from build123d import *

# Parameters (mm, degrees)
CYLINDER692_R               = 8
CYLINDER692_DEPTH           = 25
CYLINDER693_R               = 8
CYLINDER693_DEPTH           = 25
CYLINDER693_PLACEMENT_ANGLE = 225
CYLINDER695_R               = 8
CYLINDER695_DEPTH           = 25
CYLINDER694_R               = 8
CYLINDER694_DEPTH           = 25
CYLINDER694_PLACEMENT_ANGLE = 145
CYLINDER696_R               = 8
CYLINDER696_DEPTH           = 25
CYLINDER697_R               = 8
CYLINDER697_DEPTH           = 25
CYLINDER697_PLACEMENT_ANGLE = 45
CYLINDER690_R               = 8
CYLINDER690_DEPTH           = 25
CYLINDER690_ROLL_ANGLE      = 0.146073
CYLINDER690_PITCH_ANGLE     = 1.079101
CYLINDER690_PLACEMENT_ANGLE = -9.939308
CYLINDER691_R               = 8
CYLINDER691_DEPTH           = 25
CYLINDER691_PLACEMENT_ANGLE = 45
TUBE075_R                   = 38.75
TUBE075_R_2                 = 30
TUBE075_DEPTH               = 8
CHAMFER001_SIZE             = 1


with BuildPart() as obj1:
    # Cylinder692 → Cylinder692 (new body)
    with BuildSketch(Plane(origin=(-38.798949, 16.072537, 43), x_dir=(0, -1, 0), z_dir=(0, 0, 1))):
        Circle(CYLINDER692_R)
    extrude(amount=CYLINDER692_DEPTH)


with BuildPart() as obj2:
    # Cylinder693 → Cylinder693 (new body)
    with BuildSketch(Plane.XY):
        Circle(CYLINDER693_R)
    extrude(amount=CYLINDER693_DEPTH)


with BuildPart() as obj2_1:
    # Cylinder693 placement: moved
    add(obj2.part.moved(Location((-16.07, 38.8, 43))).rotate(Axis((-16.07, 38.8, 43), (0, 0, 1)), CYLINDER693_PLACEMENT_ANGLE))


with BuildPart() as obj3:
    # Cylinder695 → Cylinder695 (new body)
    with BuildSketch(Plane(origin=(16.072537, 38.798949, 43), x_dir=(-1, 0, 0), z_dir=(0, 0, 1))):
        Circle(CYLINDER695_R)
    extrude(amount=CYLINDER695_DEPTH)


with BuildPart() as obj4:
    # Cylinder694 → Cylinder694 (new body)
    with BuildSketch(Plane.XY):
        Circle(CYLINDER694_R)
    extrude(amount=CYLINDER694_DEPTH)


with BuildPart() as obj4_1:
    # Cylinder694 placement: moved
    add(obj4.part.moved(Location((34.63, 22.64, 43.6))).rotate(Axis((34.63, 22.64, 43.6), (0, 0, 1)), CYLINDER694_PLACEMENT_ANGLE))


with BuildPart() as obj5:
    # Cylinder696 → Cylinder696 (new body)
    with BuildSketch(Plane(origin=(38.798949, -16.072537, 43), x_dir=(0, 1, 0), z_dir=(0, 0, 1))):
        Circle(CYLINDER696_R)
    extrude(amount=CYLINDER696_DEPTH)


with BuildPart() as obj6:
    # Cylinder697 → Cylinder697 (new body)
    with BuildSketch(Plane.XY):
        Circle(CYLINDER697_R)
    extrude(amount=CYLINDER697_DEPTH)


with BuildPart() as obj6_1:
    # Cylinder697 placement: moved
    add(obj6.part.moved(Location((16.07, -38.8, 43))).rotate(Axis((16.07, -38.8, 43), (0, 0, 1)), CYLINDER697_PLACEMENT_ANGLE))


with BuildPart() as obj7:
    # Cylinder690 → Cylinder690 (new body)
    with BuildSketch(Plane.XY):
        Circle(CYLINDER690_R)
    extrude(amount=CYLINDER690_DEPTH)


with BuildPart() as obj7_1:
    # Cylinder690 roll: moved
    add(obj7.part.rotate(Axis((0, 0, 0), (1, 0, 0)), CYLINDER690_ROLL_ANGLE))


with BuildPart() as obj7_2:
    # Cylinder690 pitch: moved
    add(obj7_1.part.rotate(Axis((0, 0, 0), (0, 1, 0)), CYLINDER690_PITCH_ANGLE))


with BuildPart() as obj7_3:
    # Cylinder690 placement: moved
    add(obj7_2.part.moved(Location((-21.748471, -35.690226, 43.196026))).rotate(Axis((-21.748471, -35.690226, 43.196026), (0, 0, 1)), CYLINDER690_PLACEMENT_ANGLE))


with BuildPart() as compound696:
    # Cylinder691 → Cylinder691 (new body)
    with BuildSketch(Plane.XY):
        Circle(CYLINDER691_R)
    extrude(amount=CYLINDER691_DEPTH)


with BuildPart() as compound696_1:
    # Cylinder691 placement: moved
    add(compound696.part.moved(Location((-38.8, -16.07, 43))).rotate(Axis((-38.8, -16.07, 43), (0, 0, -1)), CYLINDER691_PLACEMENT_ANGLE))

    # Compound696: union obj1, obj2, obj3, obj4, obj5, obj6, obj7
    add(obj1.part)
    add(obj2_1.part)
    add(obj3.part)
    add(obj4_1.part)
    add(obj5.part)
    add(obj6_1.part)
    add(obj7_3.part)


with BuildPart() as compound696_2:
    # Compound696 placement: moved
    add(compound696_1.part.moved(Location((0, 0, 3))))


with BuildPart() as chamfer001:
    # Tube075 → Tube075 (new body)
    with BuildSketch(Plane.XY.offset(58)):
        Circle(TUBE075_R)
        Circle(TUBE075_R_2, mode=Mode.SUBTRACT)
    extrude(amount=TUBE075_DEPTH)

    # Cut317: cut Compound696
    add(compound696_2.part, mode=Mode.SUBTRACT)

    # Chamfer001
    chamfer001_edges = [chamfer001.edges().sort_by_distance(p)[0] for p in [
        (38.534079, -4.085006, 66),
        (38.01562, 7.508338, 66),
        (27.399492, -27.401284, 66),
        (-2.751597, -38.652183, 66),
        (-29.370607, -25.277064, 66),
        (-38.75, 0.001267, 66),
        (-27.399492, 27.401284, 66),
        (0.001267, 38.75, 66),
        (24.6207, 29.922961, 66),
    ]]
    chamfer(chamfer001_edges, length=CHAMFER001_SIZE)


solid = chamfer001.part
Part model, mm, in its own coordinate system. Round coordinates to 2 decimals unless told otherwise and drop trailing zeros. Write each loop counter-clockwise with the first axis right and the second up, starting at its lowest first coordinate (ties: lowest second). Pieces come first, ordered by that corner, then holes. Notation, with made-up numbers: M -25.5,8.5 L -4.5,8.5 A22 cw -4.5,39.5 Z; hole C 85,-8.75 d7. An arc over 180 degrees is marked long. Return JSON: item names as keys, results as strings. Group by question number.
(1) Pin check, flat tips, straight feed: pin 1 Ø3 at (x, z) = (16, 63.5) entering from +Y (3 decimals); pin 2 Ø1 at (x, z) = (24, 62) entering from +Y; pin 3 Ø1 at (y, z) = (-4.5, 64) entering from -X. Stop position of each tip, or through.
(2) Saw through at D-D on y = -16. Write the cut outline in (x, z), then the cut area to 3 significant figures.
(3) Saw through at C-C on y = 17.5. Write the cut outline in (x, z).
(4) Saw through at A-A on y = 0. Write the cut outline in (x, z).
(5) Drill centre lines: probe 1 along Y at (x, z) = (0, 60.75); probe 2 along X at (y, z) = (31.5, 60); probe 3 along X at (y, z) = (-32, 65). Where is each one in solid material? Low to high.
(6) Two-plate mould, pull along X, no slides. Class faces 1 (the face through (24.31, 29.52, 65.51)), 2 (the face through (-17.25, -28.98, 61.92)), 3 (the face through (12.901, 31.454, 61.944)), 4 (the face through (-2.831, -37.915, 65.729)): +X half, -X half, draft (parallel to the pull), parting line (faces both ways), or undercut.
Returned:
{
 "1": {"pin 1": "y = 30.955", "pin 2": "y = 30.81", "pin 3": "x = -38.54"},
 "2": {"outline": "M -30.8,58 L -25.38,58 L -25.38,66 L -30.8,66 Z; M 25.38,58 L 30.8,58 L 30.8,66 L 25.38,66 Z", "area": "86.8 mm²"},
 "3": {"outline": "M -30.93,58 L -24.37,58 L -24.37,66 L -30.93,66 Z; M 24.37,58 L 28.5,58 L 28.5,66 L 24.37,66 Z"},
 "4": {"outline": "M -38.75,58 L -30,58 L -30,66 L -37.75,66 L -38.75,65 Z; M 30,58 L 38.75,58 L 38.75,65 L 37.75,66 L 30,66 Z"},
 "5": {"probe 1": "-38.75 to -30, 30 to 38.75", "probe 2": "-22.57 to -19.34, -12.8 to 12.8, 19.35 to 22.57", "probe 3": "-14.37 to 11.86, 20.28 to 21.85"},
 "6": {"face 1": "+X half", "face 2": "undercut", "face 3": "undercut", "face 4": "parting line"}
}
